For this review, take the finished solid that the model builds, in its own axes (mm). Face numbers are marked on the shaded views. Give positions to 0.01 mm unless a question says otherwise; leave off trailing zeros. Loops run counter-clockwise (first coordinate to the right, second up) from the corner with the lowest first, then second, coordinate; pieces in that order, holes last. Notation, with made-up numbers: (0.5, 77) -> (35.5, 77) arc R36 ccw to (35.5, 113) -> close; hole circle Ø4 at (1.5, -13.75). An arc over 180 degrees is marked (long way). One line per question, with ' | ' between items. Start each with the question number.
(1) Wall thickness on probe 1 along X at (y, z) = (-9.5, 48.5); probe 2 along Y at (x, z) = (-39.5, 12); probe 3 along Z at (x, y) = (-19, -20): over which ranges is each line inside the solid? List them lowest first.
(2) Insertion check: P1, Ø20.5, axis at x = -36, z = 58.5, coming from the -Y side; P2, Ø6, axis at y = -25.5, z = 52.5, coming from the +X side; P3, Ø1, axis at x = -47, y = -20.5, coming from the -Z side; P4, Ø10, axis at y = -8.5, z = 47.5, coming from the -X side. Each pin has a flat end and moves straight along its axis. Give the tip position at first contact, or say it passes through.
(3) Consider section B-B (x = -37). Write out the cut boundary in (y, z), and give its area (3 significant figures).
(4) Consider section A-A (y = -10.5). Write out the cut boundary in (x, z).
(5) Consider section C-C (z = 64.5). Write out the cut boundary in (x, y), and give its area (3 significant figures).
(6) Draft analysis for pull direction Z (two halves, no side actions). For the marked faces 1, 2 and 3, state which applies: +Z half, -Z half, draft (parallel to the pull), parting line (faces both ways), or undercut.
(7) Consider section D-D (y = -24). Write out the cut boundary in (x, z), and give its area (3 significant figures).
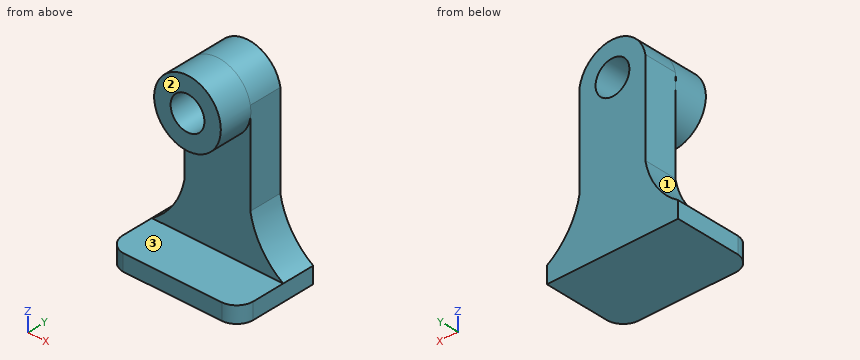
from build123d import *

# Parameters (mm, degrees)
F0_W      = 50.8
F0_H      = 6.35
F1_DEPTH  = 31.75
F2_W      = 50.8
F2_H      = 69.85
F3_DEPTH  = 12.7
F4_W      = 12.7
F4_H      = 69.85
F5_DEPTH  = 25.4
F7_DEPTH  = 12.7
F9_DEPTH  = 12.701
F10_R     = 12.888436
F11_DEPTH = 12.7
F12_R     = 6.538436
F13_DEPTH = 25.401
F15_DEPTH = 25.4
F17_DEPTH = 25.4


with BuildPart() as f1:
    # F0 (on Front) → F1 (new body)
    with BuildSketch(Plane.XZ):
        with Locations((-40.683051, 3.175)):
            Rectangle(F0_W, F0_H)
    extrude(amount=F1_DEPTH)

    # F2 (on face) → F3 (join)
    with BuildSketch(Plane(origin=(0, 0, 0), x_dir=(-1, 0, 0), z_dir=(0, 1, 0))):
        with Locations((40.683051, 41.275)):
            Rectangle(F2_W, F2_H)
    extrude(amount=-F3_DEPTH)

    # F4 (on face) → F5 (cut)
    with BuildSketch(Plane.XZ.offset(12.7)):
        with Locations((-59.733051, 41.275)):
            Rectangle(F4_W, F4_H)
        with Locations((-21.633051, 41.275)):
            Rectangle(F4_W, F4_H)
    extrude(amount=-F5_DEPTH, mode=Mode.SUBTRACT)

    # F6 (on face) → F7 (join)
    with BuildSketch(Plane(origin=(0, 0, 0), x_dir=(-1, 0, 0), z_dir=(0, 1, 0))):
        with BuildLine():
            ThreePointArc((27.983051, 25.4), (23.619413, 14.550759), (15.283051, 6.35))
            Line((15.283051, 6.35), (27.983051, 6.35))
            Line((27.983051, 6.35), (27.983051, 25.4))
        make_face()
        with BuildLine():
            Line((53.383051, 6.35), (66.083051, 6.35))
            ThreePointArc((66.083051, 6.35), (57.741785, 14.547489), (53.383051, 25.4))
            Line((53.383051, 25.4), (53.383051, 6.35))
        make_face()
    extrude(amount=-F7_DEPTH)

    # F8 (on face) → F9 (cut, through all)
    with BuildSketch(Plane.XZ.offset(12.7)):
        with BuildLine():
            ThreePointArc((-53.383051, 61.541711), (-40.683051, 72.234292), (-27.983051, 61.541711))
            Line((-27.983051, 61.541711), (-27.983051, 76.2))
            Line((-27.983051, 76.2), (-53.383051, 76.2))
            Line((-53.383051, 76.2), (-53.383051, 61.541711))
        make_face()
    extrude(amount=-F9_DEPTH, mode=Mode.SUBTRACT)

    # F10 (on face) → F11 (join)
    with BuildSketch(Plane.XZ.offset(12.7)):
        with Locations((-40.683051, 59.345856)):
            Circle(F10_R)
    extrude(amount=F11_DEPTH)

    # F12 (on face) → F13 (cut, through all)
    with BuildSketch(Plane.XZ.offset(25.4)):
        with Locations((-40.683051, 59.345856)):
            Circle(F12_R)
    extrude(amount=-F13_DEPTH, mode=Mode.SUBTRACT)

    # F14 (on face) → F15 (cut)
    with BuildSketch(Plane.XY.offset(6.35)):
        with BuildLine():
            ThreePointArc((-15.283051, -25.4), (-17.173864, -29.859187), (-21.633051, -31.75))
            Line((-21.633051, -31.75), (-15.283051, -31.75))
            Line((-15.283051, -31.75), (-15.283051, -25.4))
        make_face()
    extrude(amount=-F15_DEPTH, mode=Mode.SUBTRACT)

    # F16 (on face) → F17 (cut)
    with BuildSketch(Plane.XY.offset(6.35)):
        with BuildLine():
            ThreePointArc((-59.733051, -31.75), (-64.062729, -29.729678), (-66.083051, -25.4))
            Line((-66.083051, -25.4), (-66.083051, -31.75))
            Line((-66.083051, -31.75), (-59.733051, -31.75))
        make_face()
    extrude(amount=-F17_DEPTH, mode=Mode.SUBTRACT)


solid = f1.part
A:
1) probe 1: x = -53.38 to -27.98 | probe 2: y = -12.7 to 0 | probe 3: z = 0 to 6.35
2) P1: stops at y = -25.4 | P2: stops at x = -28.38 | P3: stops at z = 0 | P4: stops at x = -53.38
3) outline: (-31.75, 0) -> (0, 0) -> (0, 53.94) -> (-25.4, 53.94) -> (-25.4, 46.99) -> (-12.7, 46.99) -> (-12.7, 6.35) -> (-31.75, 6.35) -> close; (-25.4, 64.75) -> (0, 64.75) -> (0, 71.7) -> (-25.4, 71.7) -> close | area: 1,070 mm^2
4) outline: (-66.08, 0) -> (-15.28, 0) -> (-15.28, 6.35) arc R28.64 cw to (-27.98, 25.4) -> (-27.98, 61.54) arc R12.89 ccw to (-53.38, 61.54) -> (-53.38, 25.4) arc R28.58 cw to (-66.08, 6.35) -> close; hole circle Ø13.08 at (-40.68, 59.35)
5) outline: (-52.5, -25.4) -> (-44.71, -25.4) -> (-44.71, 0) -> (-52.5, 0) -> close; (-36.66, -25.4) -> (-28.87, -25.4) -> (-28.87, 0) -> (-36.66, 0) -> close | area: 396 mm^2
6) face 1: +Z half | face 2: draft | face 3: undercut
7) outline: (-66.08, 0) -> (-15.28, 0) -> (-15.28, 6.35) -> (-66.08, 6.35) -> close; circle Ø25.78 at (-40.68, 59.35); hole circle Ø13.08 at (-40.68, 59.35) | area: 710 mm^2
